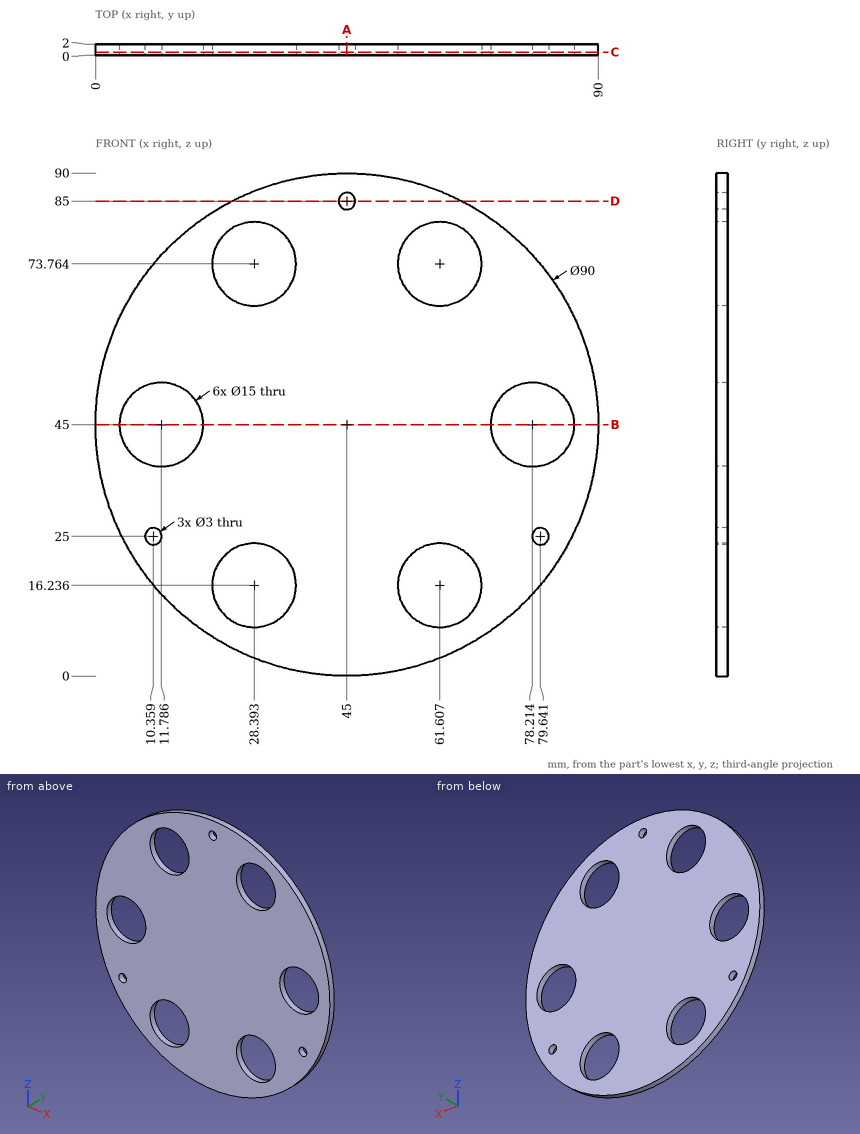
Job drawing, mm, ordinate dimensions from the low corner. One solid piece. Coordinates: 2 decimals unless noted, no trailing zeros. Loops run counter-clockwise (first coordinate to the right, second up) from the corner with the lowest first, then second, coordinate; pieces in that order, holes last. Notation, with made-up numbers: (58, 37.25) -> (66, 37.25) arc R9 ccw to (66, 54.25) -> close; hole circle Ø9 at (45, 33). An arc over 180 degrees is marked (long way). One line per item, written item: value.
1. Slice it at B-B on z = 45. Write the cut outline in (x, y), and give its area (3 significant figures).
Answers:
outline: (0, 0) -> (4.29, 0) -> (4.29, 2) -> (0, 2) -> close; (19.29, 0) -> (70.71, 0) -> (70.71, 2) -> (19.29, 2) -> close; (85.71, 0) -> (90, 0) -> (90, 2) -> (85.71, 2) -> close
area: 120 mm^2
2. Drill centre lines: line 1 (X direction, y = 1.9, z = 39); line 2 (X direction, y = 0.85, z = 38.5) (1 decimal); line 3 (Z direction, x = 66, y = 1.35) (1 decimal). Where is each one in solid material? Low to high. Write a range as [from, to].
Answers:
line 1: x = [0.4, 7.29], [16.29, 73.71], [82.71, 89.6]
line 2: x = [0.5, 8], [15.5, 74.5], [82, 89.5]
line 3: z = [5.2, 10.2], [22.3, 67.7], [79.8, 84.8]
3. Slice it at A-A on x = 45. Write the cut outline in (y, z), and give its area (3 significant figures).
Answers:
outline: (0, 0) -> (2, 0) -> (2, 83.5) -> (0, 83.5) -> close; (0, 86.5) -> (2, 86.5) -> (2, 90) -> (0, 90) -> close
area: 174 mm^2
4. Slice it at D-D on z = 85. Write the cut outline in (x, y).
Answers:
outline: (24.38, 0) -> (43.5, 0) -> (43.5, 2) -> (24.38, 2) -> close; (46.5, 0) -> (65.62, 0) -> (65.62, 2) -> (46.5, 2) -> close
5. Slice it at C-C on y = 0.55. Give the number of separate pieces and of enclosed holes in the cut face, and give its area (3 significant figures).
Answers:
separate pieces: 1
enclosed holes: 9
area: 5,280 mm^2
6. Flat gauge pins, fed straight in: P1, Ø19.5, axis at x = 61.61, z = 16.24, coming from the +Y side; P2, Ø1, axis at x = 19.5, y = 2, coming from the -Z side. Where does each tip first touch, or does it go through?
Answers:
P1: stops at y = 2
P2: stops at z = 7.58
